Design review of the part built by this model. Coordinates are the model's own, in mm. Give positions to 0.01 mm unless a question says otherwise; leave off trailing zeros. Order: outer loops, then holes, each group sorted by start corner. A loop starts at its lowest first (then second) coordinate and runs counter-clockwise, first axis right, second up. Notation, with made-up numbers: (76.25, -30) -> (108.25, -30) arc R24 cw to (108.25, -8) -> close; hole circle Ø8 at (5, 8.25). An arc over 180 degrees is marked (long way). One line per item, written item: value.
from build123d import *

# Parameters (mm, degrees)
CROQUIS1_R              = 38.99
CROQUIS1_R_2            = 37.79
SALIENTE_EXTRUIR1_DEPTH = 250
CROQUIS3_R              = 5
CORTAR_EXTRUIR1_DEPTH   = 39.99
MATRIZC4_COUNT          = 2
MATRIZC4_ANGLE          = 90
CROQUIS4_R              = 2
CORTAR_EXTRUIR2_DEPTH   = 39.9900001
MATRIZC5_COUNT          = 2
MATRIZC5_ANGLE          = 90


with BuildPart() as part:
    # Croquis1 → Saliente-Extruir1 (new body, symmetric)
    with BuildSketch(Plane(origin=(0, 0, 0), x_dir=(0, 0, -1), z_dir=(1, 0, 0))):
        Circle(CROQUIS1_R)
        Circle(CROQUIS1_R_2, mode=Mode.SUBTRACT)
    extrude(amount=SALIENTE_EXTRUIR1_DEPTH, both=True)

    # Croquis3 → Cortar-Extruir1 (cut, symmetric)
    with BuildSketch(Plane.XY):
        with Locations((10, 0)):
            Circle(CROQUIS3_R)
    cortar_extruir1 = extrude(amount=CORTAR_EXTRUIR1_DEPTH, both=True, mode=Mode.SUBTRACT)

    # MatrizC4: Cortar-Extruir1 ×2 about axis
    matrizc4_axis = Axis((250, 0, 0), (1, 0, 0))
    for i in range(1, MATRIZC4_COUNT):
        add(cortar_extruir1.rotate(matrizc4_axis, i * MATRIZC4_ANGLE / (MATRIZC4_COUNT - 1)), mode=Mode.SUBTRACT)

    # Croquis4 → Cortar-Extruir2 (cut, symmetric)
    with BuildSketch(Plane.XY):
        with Locations((223, 0)):
            Circle(CROQUIS4_R)
    cortar_extruir2 = extrude(amount=CORTAR_EXTRUIR2_DEPTH, both=True, mode=Mode.SUBTRACT)

    # MatrizC5: Cortar-Extruir2 ×2 about axis
    matrizc5_axis = Axis((250, 0, 0), (1, 0, 0))
    for i in range(1, MATRIZC5_COUNT):
        add(cortar_extruir2.rotate(matrizc5_axis, i * MATRIZC5_ANGLE / (MATRIZC5_COUNT - 1)), mode=Mode.SUBTRACT)


solid = part.part
Item 1: To check wall thickness, follow line 1 along X through (y, z) = (38.6, 0); line 2 along Y through (x, z) = (-70, 0); line 3 along Z through (x, y) = (-193, -1.5). State the ranges of each line that lie inside material, in increasing order. Write a range as from..to.
Returned:
line 1: -250..5, 15..221, 225..250
line 2: -38.99..-37.79, 37.79..38.99
line 3: -38.96..-37.76, 37.76..38.96
Item 2: Clearance check with flat-ended pins moving along their axes: P1, Ø5, axis at x = 171, y = -14, coming from the -Z side; P2, Ø10, axis at x = -164.5, z = -13.5, coming from the +Y side; P3, Ø12, axis at x = 164, z = -29, coming from the -Y side. State where each tip first meets the part, or that it passes through.
Returned:
P1: z = -37.26
P2: y = 38.05
P3: y = -31.48
Item 3: Add section A-A on z = 11.5. Give the boundary of the cut face in (x, y), plus the area to 3 significant figures.
Returned:
outline: (-250, -37.26) -> (250, -37.26) -> (250, -36) -> (-250, -36) -> close; (-250, 36) -> (250, 36) -> (250, 37.26) -> (-250, 37.26) -> close
area: 1,260 mm²
Item 4: Add section C-C on y = -31. Give the boundary of the cut face in (x, z), plus the area to 3 significant figures.
Returned:
outline: (-250, -23.65) -> (250, -23.65) -> (250, -21.61) -> (-250, -21.61) -> close; (-250, 21.61) -> (250, 21.61) -> (250, 23.65) -> (-250, 23.65) -> close
area: 2,040 mm²
Item 5: Draft analysis for pull direction Z (two halves, no side actions). For faces 1 (the cylindrical face through (12.307, 38.213, -4.436)), 2 (the flat face through (-250, 20.4, 32)), 3 (the cylindrical face through (3.5, 38.658, 5.076)), state which applies: pulls with the +Z half, pulls with the -Z half, needs draft (parallel to the pull), parting line crosses it, or undercut.
Returned:
face 1: undercut
face 2: needs draft
face 3: parting line crosses it
Item 6: Add section D-D on x = -157. Give the boundary of the cut face in (y, z).
Returned:
outline: circle Ø77.98 at (0, 0); hole circle Ø75.58 at (0, 0)
Item 7: Add section B-B on x = 10. Give the boundary of the cut face in (y, z), plus the area to 3 significant figures.
Returned:
outline: (-38.67, -5) arc R38.99 ccw to (-5, -38.67) -> (-5, -37.46) arc R37.79 cw to (-37.46, -5) -> close; (-38.67, 5) -> (-37.46, 5) arc R37.79 cw to (-5, 37.46) -> (-5, 38.67) arc R38.99 ccw to start; (5, -38.67) arc R38.99 ccw to (38.67, -5) -> (37.46, -5) arc R37.79 cw to (5, -37.46) -> close; (5, 37.46) arc R37.79 cw to (37.46, 5) -> (38.67, 5) arc R38.99 ccw to (5, 38.67) -> close
area: 241 mm²
